Work out the finished part from the listing and answer in its coordinate system (mm). Round coordinates to 2 decimals unless told otherwise and drop trailing zeros. Loops run counter-clockwise (first coordinate to the right, second up) from the corner with the lowest first, then second, coordinate; pieces in that order, holes last.
```python
from build123d import *

# Parameters (mm, degrees)
F1_DEPTH = 12.7
F3_D     = 19.05
F5_D     = 6.5278
F5_DEPTH = 19.05
F5_TIP   = 1.9611489744


# Not quite as in the source:
# - a feature names something its author has since deleted; it is built from what else it names


with BuildPart() as f1:
    # F0 (on Top) → F1 (new body)
    with BuildSketch(Plane.XY):
        with BuildLine():
            Line((38.1, 1073.25354091), (12.7, 1073.25354091))
            ThreePointArc((12.7, 1073.25354091), (3.7197438789, 1069.5337970311), (0, 1060.55354091))
            Line((0, 1060.55354091), (0, 57.25354091))
            Line((0, 57.25354091), (19.05, 57.25354091))
            Line((19.05, 57.25354091), (19.05, 863.70354091))
            ThreePointArc((19.05, 863.70354091), (20.9098719395, 868.1936689706), (25.4, 870.05354091))
            Line((25.4, 870.05354091), (44.45, 870.05354091))
            ThreePointArc((44.45, 870.05354091), (48.9401280605, 871.9134128495), (50.8, 876.40354091))
            Line((50.8, 876.40354091), (50.8, 1060.55354091))
            ThreePointArc((50.8, 1060.55354091), (47.0802561211, 1069.5337970311), (38.1, 1073.25354091))
        make_face()
    extrude(amount=F1_DEPTH)

    # F3 (through all)
    with Locations(Plane.XY.offset(12.7)):
        with Locations((50.8, 1047.85354091), (50.8, 895.45354091)):
            Hole(F3_D / 2)

    # F5
    with Locations(Plane.YZ.offset(50.8)):
        with Locations((1016.10354091, 6.35), (927.20354091, 6.35)):
            Hole(F5_D / 2, depth=F5_DEPTH)
            with Locations((0, 0, -(F5_DEPTH + F5_TIP / 2))):  # 118° drill point
                Cone(0, F5_D / 2, F5_TIP, mode=Mode.SUBTRACT)


solid = f1.part
```
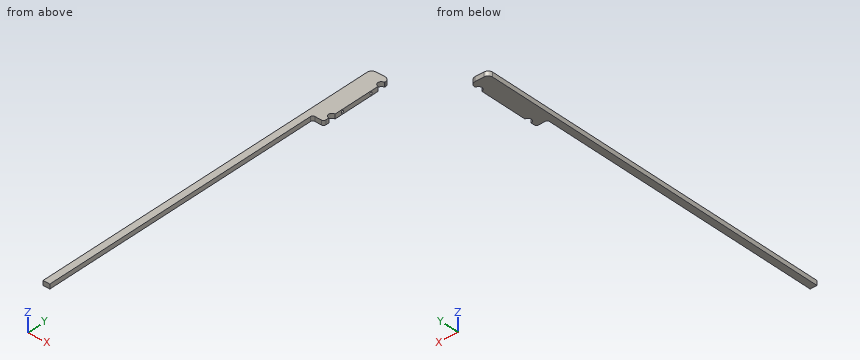
1. Find section A-A (y = 748.5). Write down the section's boundary in (x, z), then the cut area to 3 significant figures.
Answer key:
outline: (0, 0) - (19.05, 0) - (19.05, 12.7) - (0, 12.7) - close
area: 242 mm2
2. Consider probe 1 along Y at (x, z) = (39.5, 6.35); probe 2 along Y at (x, z) = (36, 6.35); probe 3 along Y at (x, z) = (42, 6.35). Determine where each line is inside the solid, lowest interval first.
Answer key:
probe 1: y = 870.05 to 923.94, 930.47 to 1012.84, 1019.37 to 1073.18
probe 2: y = 870.05 to 923.94, 930.47 to 1012.84, 1019.37 to 1073.25
probe 3: y = 870.05 to 891.81, 899.1 to 923.94, 930.47 to 1012.84, 1019.37 to 1044.21, 1051.5 to 1072.64
3. Given pin 1 (4 mm diameter, centred on x = 33.5, z = 6, fed in from -Y); pin 2 (6.5 mm diameter, centred on y = 614.5, z = 5.5, fed in from +X), each flat-ended and moving along its own axis, determine where each tip first touches the part or whether it passes through.
Answer key:
pin 1: stops at y = 870.05
pin 2: stops at x = 19.05
